Autodesk Inventor part; units mm, degrees
ref_plane "YZ Plane" through (0, 0, 0) normal (1, 0, 0) x (0, 1, 0)
ref_plane "XZ Plane" through (0, 0, 0) normal (0, 1, 0) x (-1, 0, 0)
ref_plane "XY Plane" through (0, 0, 0) normal (0, 0, 1) x (1, 0, 0)
sketch "Sketch1" plane through (0, 0, 0) normal (0, 0, 1) x (1, 0, 0)
  line L0 (0, 0) -> (129.73, 0)
  line L1 (129.73, 0) -> (129.73, 99.25)
  line L2 (129.73, 99.25) -> (0, 99.25)
  line L3 (0, 99.25) -> (0, 0)
  dimension "d0" = 129.73
  dimension "d1" = 99.25
extrude "Extrusion1" add sketch "Sketch1" along normal blind 5.7658
fillet "Fillet1" radius 3.175 4 edges at (129.73, 99.25, 2.8829) (0, 99.25, 2.8829) (0, 0, 2.8829) (129.73, 0, 2.8829)
sketch "Sketch2" plane through (0, 0, 5.7658) normal (0, 0, 1) x (1, 0, 0)
  circle A0 centre (7.62, 91.63) radius 2.7559
  circle A1 centre (122.11, 91.63) radius 2.7559
  circle A2 centre (122.11, 7.62) radius 2.7559
  circle A3 centre (7.62, 7.62) radius 2.7559
  line L0 (0, 96.075) -> (0, 3.175)
  line L1 (126.555, 99.25) -> (3.175, 99.25)
  line L2 (129.73, 3.175) -> (129.73, 96.075)
  line L3 (3.175, 0) -> (126.555, 0)
  point P0 (0, 0)
  dimension "d5" = 7.62
  dimension "d6" = 7.62
  dimension "d7" = 7.62
  dimension "d8" = 7.62
  dimension "d9" = 7.62
  dimension "d10" = 7.62
  dimension "d11" = 5.5118
  dimension "d12" = 5.5118
  dimension "d13" = 5.5118
  dimension "d14" = 7.62
  dimension "d15" = 7.62
  dimension "d16" = 5.5118
extrude "Extrusion2" cut sketch "Sketch2" against normal through all
properties part number "PowerBoardCaseCover" material "Polycarbonate, Clear"
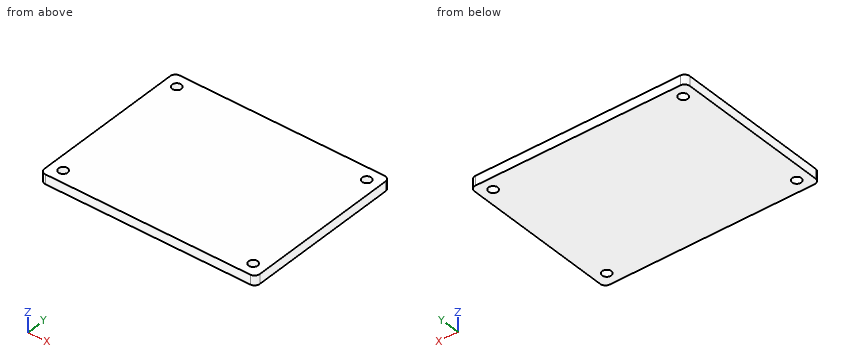
Read the model definition and answer for the solid it produces. Units are mm, in the model's axes. Give positions to 0.01 mm unless a question says otherwise; leave off trailing zeros. Order: outer loops, then holes, each group sorted by start corner. A loop starts at its lowest first (then second) coordinate and runs counter-clockwise, first axis right, second up.
(1) Straight lines are drawn through the part: L1, parallel to Y at x = 122.11, z = 2.8; L2, parallel to Y at x = 123, z = 1.25. For each, find the intervals that lie inside material, in ascending order.
(2) Find section B-B (x = 122.11). Give the vertices of the cut face in (y, z).
(3) Find section A-A (y = 7.62). Give the vertices of the cut face in (x, z), plus the area to 3 significant figures.
Result sheet:
1. L1: y = 0 to 4.86, 10.38 to 88.87, 94.39 to 99.25
1. L2: y = 0 to 5.01, 10.23 to 89.02, 94.24 to 99.25
2. outline: (0, 0) - (4.86, 0) - (4.86, 5.77) - (0, 5.77) - close; (10.38, 0) - (88.87, 0) - (88.87, 5.77) - (10.38, 5.77) - close; (94.39, 0) - (99.25, 0) - (99.25, 5.77) - (94.39, 5.77) - close
3. outline: (0, 0) - (4.86, 0) - (4.86, 5.77) - (0, 5.77) - close; (10.38, 0) - (119.35, 0) - (119.35, 5.77) - (10.38, 5.77) - close; (124.87, 0) - (129.73, 0) - (129.73, 5.77) - (124.87, 5.77) - close
3. area: 684 mm2
